Can you work these out from the model? Positions are in its coordinate system, mm. Face numbers are marked on the shaded views. Coordinates: 2 decimals unless noted, no trailing zeros. Write each loop counter-clockwise with the first axis right and the second up, starting at its lowest first coordinate (ties: lowest second). Pieces come first, ordered by that corner, then holes. Notation, with made-up numbers: (83.5, 80.5) - (140.5, 80.5) arc R19 cw to (140.5, 103.5) - close; hole circle Ø9 at (-18.5, 47.25). An arc over 180 degrees is marked (long way). Use one line per item in the form item = value. Start each with the question number.
(1) If I drill on probe 1 along Y at (x, z) = (0, 10); probe 2 along X at (y, z) = (-17.5, 35.5); probe 3 along Y at (x, z) = (-16.5, 38.5), over which ranges is the centre line in solid material (lowest first)? Write a range as from..to.
(2) If we section it at A-A on y = 0: Please give me the cut outline in (x, z), then the cut area to 3 significant figures.
(3) If we section it at C-C on z = 31.5: Please give me the cut outline in (x, y), then the cut area to 3 significant figures.
(4) If we section it at B-B on x = -17: Please give me the cut outline in (y, z).
(5) For pin 1 Ø1.4 at (y, z) = (-21, 13.5) entering from +X; pin 2 Ø0.7 at (y, z) = (-20.5, 26) entering from -X; pin 3 Ø8 at (x, z) = (-18, 37) entering from -Y; pin 4 Ø3.5 at (x, z) = (0.5, 10.5) entering from +Y, each with a flat end and sliding along its axis, tell me the tip position at first contact or that it passes through.
(6) If we section it at D-D on x = 0: Please give me the cut outline in (y, z), then the cut area to 3 significant figures.
(7) Thinking about a two-plate mould opening in X: for the marked faces 1 and 2, which applies, pulls with the +X half, pulls with the -X half, needs draft (parallel to the pull), parting line crosses it, or undercut?
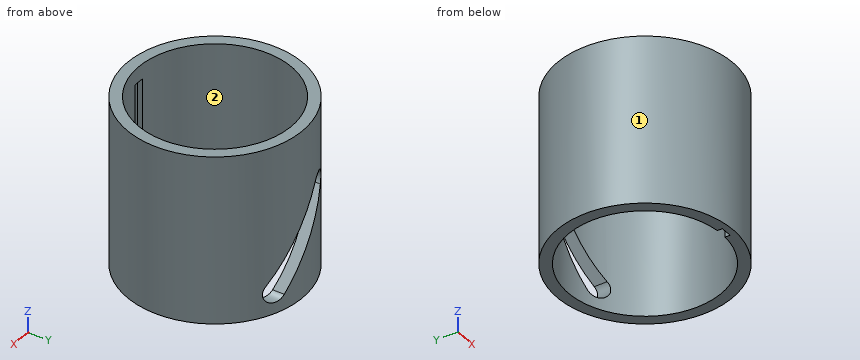
```python
from build123d import *

# Parameters (mm, degrees)
SKETCH_1_R          = 23
SKETCH_1_R_2        = 20.05
EXTRUDE_1_DEPTH     = 44
CUT_EXTRUDE_1_DEPTH = 40
SKETCH_3_W          = 3
SKETCH_3_H          = 2.5
CUT_EXTRUDE_2_DEPTH = 40


with BuildPart() as part:
    # 스케치1 → 보스-돌출1 (new body)
    with BuildSketch(Plane.XY):
        Circle(SKETCH_1_R)
        Circle(SKETCH_1_R_2, mode=Mode.SUBTRACT)
    extrude(amount=EXTRUDE_1_DEPTH)

    # 스케치2 → 컷-돌출1 (cut)
    with BuildSketch(Plane(origin=(0, 0, 0), x_dir=(1, 0, 0), z_dir=(0, 1, 0))):
        with BuildLine():
            Line((-10.470977563, -22.970475817), (5.930302333, -3.982092632))
            ThreePointArc((5.930302333, -3.982092632), (10.161651705, -3.672766774), (10.470977563, -7.904116147))
            Line((10.470977563, -7.904116147), (-5.930302333, -26.892499333))
            ThreePointArc((-5.930302333, -26.892499333), (-10.161651705, -27.20182519), (-10.470977563, -22.970475817))
        make_face()
    extrude(amount=CUT_EXTRUDE_1_DEPTH, mode=Mode.SUBTRACT)

    # 스케치3 → 컷-돌출2 (cut)
    with BuildSketch(Plane.XY):
        with Locations((0, -20.05)):
            Rectangle(SKETCH_3_W, SKETCH_3_H)
    extrude(amount=CUT_EXTRUDE_2_DEPTH, mode=Mode.SUBTRACT)


solid = part.part
```
Reported:
q1.probe_1 = -23..-21.3, 20.05..23
q1.probe_2 = -14.92..-9.79, 9.79..14.92
q1.probe_3 = -16.02..-11.39, 11.39..16.02
q2.outline = (-23, 0) - (-20.05, 0) - (-20.05, 44) - (-23, 44) - close; (20.05, 0) - (23, 0) - (23, 44) - (20.05, 44) - close
q2.area = 260 mm2
q3.outline = circle Ø46 at (0, 0); hole (-1.5, -21.3) - (1.5, -21.3) - (1.5, -19.99) arc R20.05 ccw (long way) to (-1.5, -19.99) - close
q3.area = 395 mm2
q4.outline = (-15.49, 0) - (-10.63, 0) - (-10.63, 44) - (-15.49, 44) - close; (10.63, 0) - (15.49, 0) - (15.49, 44) - (10.63, 44) - close
q5.pin_1 = 10.81
q5.pin_2 = -11.09
q5.pin_3 = -18.25
q5.pin_4 = 23
q6.outline = (-23, 0) - (-21.3, 0) - (-21.3, 40) - (-20.05, 40) - (-20.05, 44) - (-23, 44) - close; (20.05, 0) - (23, 0) - (23, 10.85) - (20.05, 10.85) - close; (20.05, 20.03) - (23, 20.03) - (23, 44) - (20.05, 44) - close
q6.area = 183 mm2
q7.face_1 = parting line crosses it
q7.face_2 = undercut
